Check sheet for the drawn part. Datum: minimum x, y, z corner. Units: mm. Coordinates: 2 decimals unless noted, no trailing zeros. Write each loop counter-clockwise with the first axis right and the second up, starting at its lowest first coordinate (ties: lowest second). Pieces come first, ordered by that corner, then holes. Notation, with made-up numbers: M 77,27.5 L 132,27.5 A21 cw 132,42.5 Z; hole C 62.5,-34 d2. An arc over 180 degrees is marked long. Answer as CSV lines item,"result". Start each with the question number.
Q1. Thickness scan on line 1 along X through (y, z) = (0.6, 14.25) (3 decimals); line 2 along Z through (x, y) = (52.5, 2.2) (3 decimals); line 3 along X through (y, z) = (3.3, 11.75) (3 decimals). Record the ranges inside material, lowest first. Write a range as from..to.
Q2. Sectioned sample at A-A, the plane z = 13.5. Record the cut outline in (x, y) (3 decimals), then the cut area to 3 significant figures.
Q3. Sectioned sample at B-B, the plane y = 3.75. Record the cut outline in (x, z) (3 decimals), then the cut area to 3 significant figures.
Q4. Sectioned sample at C-C, the plane x = 25. Record the cut outline in (y, z) (3 decimals).
Q5. Sectioned sample at D-D, the plane z = 3.5. Record the cut outline in (x, y), then the cut area to 3 significant figures.
Q6. Depth check by flat-ended pin: pin 1 Ø1.5 at (y, z) = (2, 14.5) entering from -X (3 decimals); pin 2 Ø1.5 at (x, y) = (19, 3) entering from +Z (3 decimals). Enter the tip coordinate at first touch or a pass-through.
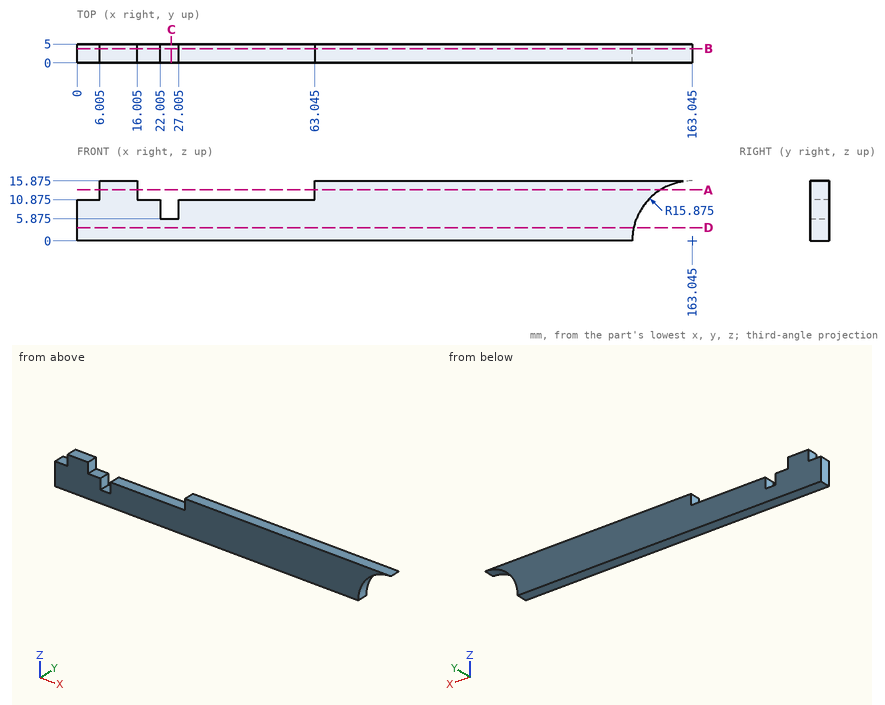
Output:
1,line 1,"x = 6.005..16.005, 63.045..156.048"
1,line 2,"z = 0..10.875"
1,line 3,"x = 6.005..16.005, 63.045..152.37"
2,outline,"M 6.005,0 L 16.005,0 L 16.005,5 L 6.005,5 Z; M 63.045,0 L 154.692,0 L 154.692,5 L 63.045,5 Z"
2,area,"508 mm^2"
3,outline,"M 0,0 L 147.17,0 A15.875 cw 163.045,15.875 L 63.045,15.875 L 63.045,10.875 L 27.005,10.875 L 27.005,5.875 L 22.005,5.875 L 22.005,10.875 L 16.005,10.875 L 16.005,15.875 L 6.005,15.875 L 6.005,10.875 L 0,10.875 Z"
3,area,"2,100 mm^2"
4,outline,"M 0,0 L 5,0 L 5,5.875 L 0,5.875 Z"
5,outline,"M 0,0 L 147.56,0 L 147.56,5 L 0,5 Z"
5,area,"738 mm^2"
6,pin 1,"stops at x = 6.005"
6,pin 2,"stops at z = 10.875"
